Autodesk Inventor part; units mm, degrees
ref_plane "YZ Plane" through (0, 0, 0) normal (1, 0, 0) x (0, 1, 0)
ref_plane "XZ Plane" through (0, 0, 0) normal (0, 1, 0) x (-1, 0, 0)
ref_plane "XY Plane" through (0, 0, 0) normal (0, 0, 1) x (1, 0, 0)
sketch "草圖1" plane through (0, 0, 0) normal (1, 0, 0) x (0, 1, 0)
  line L0 (0, -28.5) -> (61, -28.5)
  line L1 (61, -28.5) -> (72, -34.8304)
  line L2 (72, -34.8304) -> (136, -34.8304)
  line L3 (136, -30.6704) -> (73.1116, -30.6704)
  line L4 (73.1116, -30.6704) -> (62.1116, -24.34)
  line L5 (62.1116, -24.34) -> (0, -24.34)
  line L6 (136, -34.8304) -> (136, -30.6704)
  line L7 (0, -28.5) -> (0, -24.34)
  line L8 (-27.2, 0) -> (163.2, 0)
  point P0 (0, 0)
  dimension "d1" = 61
  dimension "d4" = 64
  dimension "d5" = 28.5
  dimension "d6" = 11
  dimension "d7" = 4.16
revolve "迴轉1" add sketch "草圖1" angle 360 about axis through (0, -10, 0) along (0, 1, 0)
sketch "草圖2" plane through (0, 0, 0) normal (1, 0, 0) x (0, 1, 0)
  line L0 (72, -34.8304) -> (72, 34.8304)
  line L1 (72, 6.45) -> (90.9, 6.45)
  line L2 (90.9, 6.45) -> (90.9, -6.45)
  line L3 (90.9, -6.45) -> (72, -6.45)
  line L4 (72, -6.45) -> (72, 6.45)
  point P0 (0, 0)
  point P1 (72, 0)
  dimension "d9" = 18.9
  dimension "d10" = 12.9
extrude "擠出1" cut sketch "草圖2" along normal through all
sketch "草圖3" plane through (0, 0, 0) normal (1, 0, 0) x (0, 1, 0)
  line L0 (72, -6.45) -> (72, 6.45)
  line L1 (72, 6.45) -> (72, -6.45)
  line L2 (61, -28.5) -> (61, 28.5)
  line L3 (61, -28.5) -> (72, -34.8304)
  line L4 (72, -34.8304) -> (72, 34.8304)
  line L5 (61, 28.5) -> (72, 34.8304)
  line L6 (61, -28.5) -> (61, 28.5)
  line L7 (72, -21.3304) -> (61, -15)
  line L8 (72, 21.3304) -> (61, 15)
  point P0 (0, 0)
  point P1 (61, 0)
  point P2 (61, 0)
  dimension "d17" = 15
  dimension "d18" = 15
extrude "擠出2" cut sketch "草圖3" against normal through all contours L4 L7 L2 L8 L0
pattern_circular "環形陣列1" count 3 over 360 about axis through (0, -10, 0) along (0, 1, 0) of "擠出2"
properties part number "outercase"
Could you check a few things on this model? Use its own coordinates, in mm. A direction names the side the tool comes from. Give positions to 0.01 mm unless a question says otherwise; leave off trailing zeros. Loops run counter-clockwise (first coordinate to the right, second up) from the corner with the lowest first, then second, coordinate; pieces in that order, holes last. Notation, with made-up numbers: (-34, 40) -> (-16, 40) arc R20 ccw to (-16, 62) -> close; hole circle Ø7 at (32.5, -27.75). An arc over 180 degrees is marked (long way). Return JSON: item names as keys, results as strings.
Item 1: I need wall thicknesses on L1, parallel to Z at x = 0, y = 37; L2, parallel to Z at x = 0, y = 105.5. Which ranges of each line are inside material? Lowest first, please. Write a range as from..to.
Geometry results:
{"L1": "z = -28.5..-24.34, 24.34..28.5", "L2": "z = -34.83..-30.67, 30.67..34.83"}
Item 2: If we section it at C-C on x = 5.5: Count the separate pieces of the cut face and the enclosed holes in it, plus the area to 3 significant figures.
Geometry results:
{"separate pieces": "4", "enclosed holes": "0", "area": "1,060 mm²"}
Item 3: If we section it at A-A on y = 107: List the corners of the cut face in (x, z) for me.
Geometry results:
{"outline": "circle Ø69.66 at (0, 0); hole circle Ø61.34 at (0, 0)"}
Item 4: I'm going to push flat-ended pins straight in: pin 1 (2 mm diameter, centred on y = 120.5, z = 27, fed in from -X); pin 2 (1 mm diameter, centred on x = 9.5, y = 52, fed in from +Z); pin 3 (4 mm diameter, centred on x = 32.5, y = 83.5, fed in from -Z). Where does each tip first touch, or does it pass through?
Geometry results:
{"pin 1": "stops at x = -23.18", "pin 2": "stops at z = 27.04", "pin 3": "stops at z = -16.82"}
Item 5: If we section it at B-B on z = 0: List the corners of the cut face in (x, y) for me, plus the area to 3 significant figures.
Geometry results:
{"outline": "(-34.83, 72) -> (-30.03, 72) -> (-30.67, 73.11) -> (-30.67, 136) -> (-34.83, 136) -> close; (-28.5, 0) -> (-24.34, 0) -> (-24.34, 61) -> (-28.5, 61) -> close; (24.34, 0) -> (28.5, 0) -> (28.5, 61) -> (34.83, 72) -> (30.03, 72) -> (24.34, 62.11) -> close; (30.67, 90.9) -> (34.83, 90.9) -> (34.83, 136) -> (30.67, 136) -> close", "area": "1,010 mm²"}
Item 6: We'd pull the mould along Y, two halves only. Please class faces 5 (the flat face through (32, 90.9, 0)), 6 (the flat face through (-25, 61, 0)), 7 (the conical face through (31.005, 65.355, 0.214)): +Y half, -Y half, draft (parallel to the pull), parting line (faces both ways), or undercut.
Geometry results:
{"face 5": "undercut", "face 6": "+Y half", "face 7": "-Y half"}
Item 7: Which directions (+Z, -Z, +X, -X, +Y, -Y) give clear straight access to the entire face, cutting with the end or side of a thin tool? Please do faces 1 (the flat face through (-13, 0, -21)), 2 (the cylindrical face through (10.916, 30.927, -26.327)), 3 (the flat face through (32, 82, -6.45)), 4 (the cylindrical face through (-29.94, 104.12, 6.65)).
Geometry results:
{"face 1": "+Z, -Z, +X, -X, -Y", "face 2": "-Y", "face 3": "+X", "face 4": "+Y"}
